from build123d import *

# Parameters (mm, degrees)
BOSS_EXTRUDE1_DEPTH = 139.7
SKETCH2_R           = 6.35
CUT_EXTRUDE1_DEPTH  = 38.1


with BuildPart() as part:
    # Sketch1 → Boss-Extrude1 (new, symmetric)
    with BuildSketch(Plane.XY):
        Polygon((6.35, 63.5), (15.875, 53.975), (6.35, 44.45), (6.35, 0), (-6.35, 0), (-6.35, 63.5), align=None)
    extrude(amount=BOSS_EXTRUDE1_DEPTH, both=True)

    # Sketch2 → Cut-Extrude1 (cut, symmetric)
    with BuildSketch(Plane(origin=(0, 0, 0), x_dir=(0, 0, -1), z_dir=(1, 0, 0))):
        with Locations((-69.85, 25.4)):
            Circle(SKETCH2_R)
        with Locations((0, 25.4)):
            Circle(SKETCH2_R)
        with Locations((69.85, 25.4)):
            Circle(SKETCH2_R)
    extrude(amount=CUT_EXTRUDE1_DEPTH, both=True, mode=Mode.SUBTRACT)


solid = part.part
Work out the finished part from the listing and answer in its coordinate system (mm). Round coordinates to 2 decimals unless told otherwise and drop trailing zeros. Loops run counter-clockwise (first coordinate to the right, second up) from the corner with the lowest first, then second, coordinate; pieces in that order, holes last. Notation, with made-up numbers: M 45,78 L 71,78 A18 ccw 71,110 Z; hole C 50,24 d2. An arc over 180 degrees is marked long. One line per question, with ' | ' between items. Start each with the question number.
(1) A cutting plane is placed at D-D on z = -105.5. Write down the section's boundary in (x, y) (3 decimals).
(2) A cutting plane is placed at B-B on y = 25.4. Write down the section's boundary in (x, z).
(3) A cutting plane is placed at C-C on x = -2.5. Write down the section's boundary in (y, z), plus the area to 3 significant figures.
(4) For a pull along Y with two mould halves and no side action, classify faces 1 (the face through (0.089, 19.766, -2.93)), 2 (the face through (11.05, 58.8, 1.96)), 3 (the face through (0, 0, 2)), 4 (the face through (6.35, 18, 2)) as released by +Y, released by -Y, zero draft, split by the parting line, or undercut.
(5) Find the intervals of material crossed by line 1 (Z direction, x = -1, y = 22); line 2 (Z direction, x = 2, y = 29.5); line 3 (Y direction, x = 0.25, z = 0), in increasing order.
(6) A cutting plane is placed at A-A on z = 69.85. Write down the section's boundary in (x, y) (3 decimals).
(7) Flat-ended cylindrical pins translate along their axes: pin 1 Ø20.5 at (y, z) = (25.4, -69.85) entering from +X; pin 2 Ø2 at (x, z) = (10, -69) entering from -Y; pin 3 Ø1.5 at (x, z) = (12, 17) entering from -Y; pin 4 Ø7.5 at (y, z) = (25.4, 0) entering from -X. Find the tip coordinate at first contact, or state that the pin passes through.
Geometry check:
1) outline: M -6.35,0 L 6.35,0 L 6.35,44.45 L 15.875,53.975 L 6.35,63.5 L -6.35,63.5 Z
2) outline: M -6.35,-139.7 L 6.35,-139.7 L 6.35,-76.2 L -6.35,-76.2 Z; M -6.35,-63.5 L 6.35,-63.5 L 6.35,-6.35 L -6.35,-6.35 Z; M -6.35,6.35 L 6.35,6.35 L 6.35,63.5 L -6.35,63.5 Z; M -6.35,76.2 L 6.35,76.2 L 6.35,139.7 L -6.35,139.7 Z
3) outline: M 0,-139.7 L 63.5,-139.7 L 63.5,139.7 L 0,139.7 Z; hole C 25.4,-69.85 d12.7; hole C 25.4,0 d12.7; hole C 25.4,69.85 d12.7 | area: 17,400 mm²
4) face 1: undercut | face 2: released by +Y | face 3: released by -Y | face 4: zero draft
5) line 1: z = -139.7 to -75.21, -64.49 to -5.36, 5.36 to 64.49, 75.21 to 139.7 | line 2: z = -139.7 to -74.7, -65 to -4.85, 4.85 to 65, 74.7 to 139.7 | line 3: y = 0 to 19.05, 31.75 to 63.5
6) outline: M -6.35,0 L 6.35,0 L 6.35,19.05 L -6.35,19.05 Z; M -6.35,31.75 L 6.35,31.75 L 6.35,44.45 L 15.875,53.975 L 6.35,63.5 L -6.35,63.5 Z
7) pin 1: stops at x = 6.35 | pin 2: stops at y = 47.1 | pin 3: stops at y = 49.35 | pin 4: passes through
